Read the model definition and answer for the solid it produces. Units are mm, in the model's axes. A direction names the side the tool comes from. Give positions to 0.01 mm unless a question says otherwise; leave off trailing zeros. Order: outer loops, then holes, each group sorted by start corner. A loop starts at its lowest first (then second) coordinate and runs counter-clockwise, first axis right, second up. Notation, with made-up numbers: (80, 64.5) -> (84, 64.5) arc R4 cw to (84, 71.5) -> close; hole circle Ø9 at (67.5, -29). An arc over 180 degrees is marked (long way). Use one line per item in the form item = value.
```python
from build123d import *

# Parameters (mm, degrees)
SKETCH1_W           = 36.068
SKETCH1_H           = 114.808
BOSS_EXTRUDE1_DEPTH = 39.878
SKETCH3_R           = 10.795
BOSS_EXTRUDE2_DEPTH = 19.05
SKETCH4_R           = 10.795
BOSS_EXTRUDE4_DEPTH = 19.05


with BuildPart() as part:
    # Sketch1 → Boss-Extrude1 (new body)
    with BuildSketch(Plane(origin=(0, 0, 0), x_dir=(1, 0, 0), z_dir=(0, 1, 0))):
        with Locations((18.034, 57.404)):
            Rectangle(SKETCH1_W, SKETCH1_H)
    extrude(amount=BOSS_EXTRUDE1_DEPTH)

    # Sketch3 → Boss-Extrude2 (add)
    with BuildSketch(Plane.ZY):
        with Locations((-21.082, 19.939)):
            Circle(SKETCH3_R)
    extrude(amount=BOSS_EXTRUDE2_DEPTH)

    # Sketch4 → Boss-Extrude4 (add)
    with BuildSketch(Plane(origin=(36.068, 0, 0), x_dir=(0, 0, -1), z_dir=(1, 0, 0))):
        with Locations((21.082, 19.939)):
            Circle(SKETCH4_R)
    extrude(amount=BOSS_EXTRUDE4_DEPTH)


solid = part.part
```
Item 1: Which of the six approach directions +Z, -Z, +X, -X, +Y, -Y give full straight-line access (tool end or side, diameter ignored) to faces 1 (the cylindrical face through (45.46, 13.37, -12.515)), 2 (the flat face through (-19.05, 20, -21)), 3 (the cylindrical face through (-9.392, 20.414, -31.867))?
Checks:
face_1 = +X
face_2 = +Z, -Z, -X, +Y, -Y
face_3 = -X
Item 2: Straight lines are drawn through the part: L1, parallel to X at y = 21.5, z = -9.5; L2, parallel to Y at x = 52, z = -15; L3, parallel to Z at x = -3, y = 14.5. For each, find the intervals that lie inside material, in ascending order. Write a range as from..to.
Checks:
L1 = 0..36.07
L2 = 11.02..28.86
L3 = -30.41..-11.76
Item 3: The part is cut by section B-B on z = -88.5. Give the vertices of the cut face in (x, y).
Checks:
outline = (0, 0) -> (36.07, 0) -> (36.07, 39.88) -> (0, 39.88) -> close
Item 4: The part is cut by section C-C on x = -4. Give the vertices of the cut face in (y, z) (3 decimals).
Checks:
outline = circle Ø21.59 at (19.939, -21.082)
Item 5: The part is cut by section A-A on y = 11. Give the vertices of the cut face in (x, z), and give its area (3 significant figures).
Checks:
outline = (-19.05, -27.13) -> (0, -27.13) -> (0, -114.81) -> (36.07, -114.81) -> (36.07, -27.13) -> (55.12, -27.13) -> (55.12, -15.03) -> (36.07, -15.03) -> (36.07, 0) -> (0, 0) -> (0, -15.03) -> (-19.05, -15.03) -> close
area = 4,600 mm²
Item 6: Given pin 1 Ø6 at (y, z) = (10, -31) entering from -X; pin 2 Ø12 at (y, z) = (16.5, -82.5) entering from +X, each flat-ended and moving along its own axis, determine where each tip first touches the part or whether it passes through.
Checks:
pin_1 = 0
pin_2 = 36.07
Item 7: The part is cut by section D-D on y = 22. Give the vertices of the cut face in (x, z).
Checks:
outline = (-19.05, -31.68) -> (0, -31.68) -> (0, -114.81) -> (36.07, -114.81) -> (36.07, -31.68) -> (55.12, -31.68) -> (55.12, -10.49) -> (36.07, -10.49) -> (36.07, 0) -> (0, 0) -> (0, -10.49) -> (-19.05, -10.49) -> close
